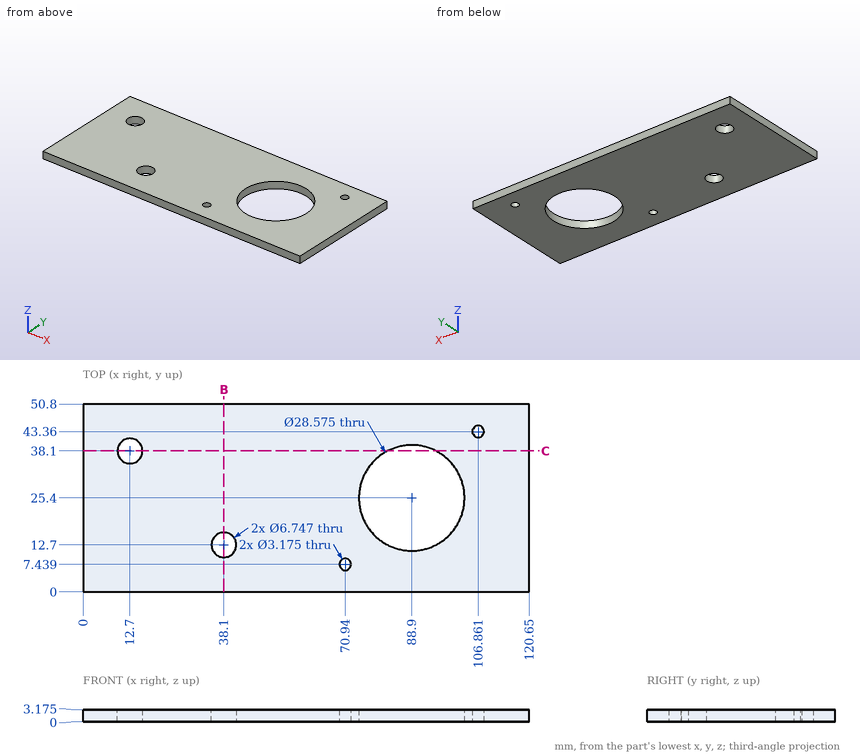
Can you work these out from the drawing? Everything is in mm from the part's minimum corner. Round coordinates to 2 decimals unless told otherwise and drop trailing zeros. Write each loop counter-clockwise with the first axis right and the second up, starting at its lowest first coordinate (ties: lowest second). Pieces come first, ordered by that corner, then holes.
1. Suppose I cut it at C-C (y = 38.1). State how many separate pieces and enclosed holes the cut face has, and give its area (3 significant figures).
2. Suppose I cut it at B-B (x = 38.1). List the corners of the cut face in (y, z) for me (1 decimal), and give its area (3 significant figures).
3. I need wall thicknesses on L1, parallel to Y at x = 88.9, z = 1.9; L2, parallel to X at y = 43.5, z = 2.1; L3, parallel to Y at x = 38.1, z = 2.4. Which ranges of each line are inside material? Lowest first, please.
4. Will this pin go through, and if not, where does the flat tip stop? pin 1 Ø23 at (x, y) = (88.9, 25.4) entering from +Z.
Answer sheet:
1. separate pieces: 3
1. enclosed holes: 0
1. area: 320 mm2
2. outline: (0, 0) - (9.3, 0) - (9.3, 3.2) - (0, 3.2) - close; (16.1, 0) - (50.8, 0) - (50.8, 3.2) - (16.1, 3.2) - close
2. area: 140 mm2
3. L1: y = 0 to 11.11, 39.69 to 50.8
3. L2: x = 0 to 105.28, 108.44 to 120.65
3. L3: y = 0 to 9.33, 16.07 to 50.8
4. pin 1: passes through
